from build123d import *

# Parameters (mm, degrees)
SKETCH3_W                    = 195
SKETCH3_H                    = 90
BASE_FLANGE1_DEPTH           = 0.76
EDGE_FLANGE1_STRIP_W         = 4.564
EDGE_FLANGE1_STRIP_H         = 0.76
EDGE_FLANGE1_STRIP_CUT_DEPTH = 90
EDGE_FLANGE1_DEPTH           = 90
EDGE_FLANGE2_STRIP_CUT_DEPTH = 90
EDGE_FLANGE2_DEPTH           = 90
EDGE_FLANGE3_STRIP_W         = 4.564
EDGE_FLANGE3_STRIP_H         = 0.76
EDGE_FLANGE3_STRIP_CUT_DEPTH = 90
EDGE_FLANGE3_DEPTH           = 90
EDGE_FLANGE6_DEPTH           = 124.238
EDGE_FLANGE7_DEPTH           = 124.238
CUT_EXTRUDE1_REACH           = 252.208


# Sheet-metal steps are written as plain solids
with BuildPart() as part:
    # Sketch3 → Base-Flange1 (new body)
    with BuildSketch(Plane(origin=(0, 0, 0), x_dir=(1, 0, 0), z_dir=(0, 1, 0))):
        with Locations((-97.5, 45)):
            Rectangle(SKETCH3_W, SKETCH3_H)
    extrude(amount=-BASE_FLANGE1_DEPTH)

    # Edge-Flange1 strip (across the edge) → Edge-Flange1 strip cut (cut)
    with BuildSketch(Plane(origin=(-195, 0, -90), x_dir=(1, 0, 0), z_dir=(0, 0, 1))):
        with Locations((-1.52, -0.38)):
            Rectangle(EDGE_FLANGE1_STRIP_W, EDGE_FLANGE1_STRIP_H)
    extrude(amount=EDGE_FLANGE1_STRIP_CUT_DEPTH, mode=Mode.SUBTRACT)

    # Edge-Flange1 section (across the edge) → Edge-Flange1 (add)
    with BuildSketch(Plane(origin=(-195, 0, -90), x_dir=(1, 0, 0), z_dir=(0, 0, 1))):
        with BuildLine():
            Line((-0.76, 0.762), (-0.76, 55))
            Line((-0.76, 55), (0, 55))
            Line((0, 55), (0, 0.762))
            ThreePointArc((0, 0.762), (0.223184633, 0.223184633), (0.762, 0))
            Line((0.762, 0), (0.762, -0.76))
            ThreePointArc((0.762, -0.76), (-0.314216521, -0.314216521), (-0.76, 0.762))
        make_face()
    extrude(amount=EDGE_FLANGE1_DEPTH)

    # Edge-Flange2 strip (across the edge) → Edge-Flange2 strip cut (cut)
    with BuildSketch(Plane(origin=(-195, 55, -90), x_dir=(-0.2588190451025146, -0.96592582628907, 0), z_dir=(0, 0, 1))):
        Polygon((-4.589327535, -2.016516504), (1.155922587, -0.477081374), (0.959220112, 0.257022254), (-4.786030009, -1.282412876), align=None)
    extrude(amount=EDGE_FLANGE2_STRIP_CUT_DEPTH, mode=Mode.SUBTRACT)

    # Edge-Flange2 section (across the edge) → Edge-Flange2 (add)
    with BuildSketch(Plane(origin=(-195, 55, -90), x_dir=(-0.2588190451025146, -0.96592582628907, 0), z_dir=(0, 0, 1))):
        with BuildLine():
            Line((-0.76, 0.993057734), (-0.76, 200))
            Line((-0.76, 200), (0, 200))
            Line((0, 200), (0, 0.993057734))
            ThreePointArc((0, 0.993057734), (0.298123791, 0.388522489), (0.959220112, 0.257022254))
            Line((0.959220112, 0.257022254), (1.155922587, -0.477081374))
            ThreePointArc((1.155922587, -0.477081374), (-0.164534895, -0.21442605), (-0.76, 0.993057734))
        make_face()
    extrude(amount=EDGE_FLANGE2_DEPTH)

    # Edge-Flange3 strip (across the edge) → Edge-Flange3 strip cut (cut)
    with BuildSketch(Plane(origin=(0, 0, 0), x_dir=(-1, 0, 0), z_dir=(0, 0, -1))):
        with Locations((-1.52, -0.38)):
            Rectangle(EDGE_FLANGE3_STRIP_W, EDGE_FLANGE3_STRIP_H)
    extrude(amount=EDGE_FLANGE3_STRIP_CUT_DEPTH, mode=Mode.SUBTRACT)

    # Edge-Flange3 section (across the edge) → Edge-Flange3 (add)
    with BuildSketch(Plane(origin=(0, 0, 0), x_dir=(-1, 0, 0), z_dir=(0, 0, -1))):
        with BuildLine():
            Line((-0.76, 0.762), (-0.76, 125))
            Line((-0.76, 125), (0, 125))
            Line((0, 125), (0, 0.762))
            ThreePointArc((0, 0.762), (0.223184633, 0.223184633), (0.762, 0))
            Line((0.762, 0), (0.762, -0.76))
            ThreePointArc((0.762, -0.76), (-0.314216521, -0.314216521), (-0.76, 0.762))
        make_face()
    extrude(amount=EDGE_FLANGE3_DEPTH)

    # Edge-Flange6 section (across the edge) → Edge-Flange6 (add)
    with BuildSketch(Plane(origin=(0, 0.762, 0.762), x_dir=(0, 0, -1), z_dir=(0, 1, 0))):
        with BuildLine():
            Line((-0.76, 0.762), (-0.76, 195.76))
            Line((-0.76, 195.76), (0, 195.76))
            Line((0, 195.76), (0, 0.762))
            ThreePointArc((0, 0.762), (0.223184633, 0.223184633), (0.762, 0))
            Line((0.762, 0), (0.762, -0.76))
            ThreePointArc((0.762, -0.76), (-0.314216521, -0.314216521), (-0.76, 0.762))
        make_face()
    extrude(amount=EDGE_FLANGE6_DEPTH)

    # Edge-Flange7 section (across the edge) → Edge-Flange7 (add)
    with BuildSketch(Plane(origin=(0, 125, -90.762), x_dir=(0, 0, 1), z_dir=(0, -1, 0))):
        with BuildLine():
            Line((-0.76, 0.762), (-0.76, 195.76))
            Line((-0.76, 195.76), (0, 195.76))
            Line((0, 195.76), (0, 0.762))
            ThreePointArc((0, 0.762), (0.223184633, 0.223184633), (0.762, 0))
            Line((0.762, 0), (0.762, -0.76))
            ThreePointArc((0.762, -0.76), (-0.314216521, -0.314216521), (-0.76, 0.762))
        make_face()
    extrude(amount=EDGE_FLANGE7_DEPTH)

    # Sketch29 → Cut-Extrude1 (cut, up to next)
    with BuildSketch(Plane.XY.offset(1.522), mode=Mode.PRIVATE) as cut_extrude1_sk1:
        Polygon((-195.76, 53.762), (-0.762, 0.762), (-195.76, 0.762), align=None)
    cut_extrude1_tool1 = extrude(cut_extrude1_sk1.sketch, amount=-CUT_EXTRUDE1_REACH, mode=Mode.PRIVATE) & part.part
    add(cut_extrude1_tool1.solids().sort_by_distance((-130.760667, 18.428667, 1.522))[0], mode=Mode.SUBTRACT)


solid = part.part
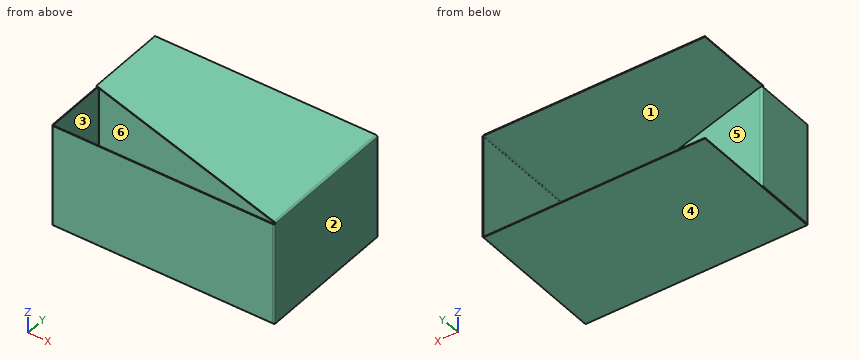
Design review of the part built by this model. Coordinates are the model's own, in mm. Face numbers are marked on the shaded views. A direction names the side the tool comes from. Round coordinates to 2 decimals unless told otherwise and drop trailing zeros. Write each loop counter-clockwise with the first axis right and the second up, starting at its lowest first coordinate (ties: lowest second). Pieces come first, ordered by that corner, then holes.
Item 1: For the marked faces 4, 5 and 6, list the 3-axis set-ups (+Z, -Z, +X, -X, +Y, -Y) from which the entire face can be reached by the end or side of a thin tool; tool diameter is ignored.
Item 2: Consider section B-B on x = -20. Give the boundary of the cut face in (y, z), and give its area (3 significant figures).
Item 3: For pin 1 Ø17 at (x, y) = (-124.5, 18.5) entering from +Z; pin 2 Ø1.5 at (x, z) = (-137, -80.5) entering from +Y; pin 3 Ø0.8 at (x, z) = (0, 0.5) entering from -Y, all flat-tipped, find the tip position at first contact; note any pin that passes through.
Item 4: Draft analysis for pull direction X (two halves, no side actions). For the marked faces 1, 2 and 3, state which applies: released by +X, released by -X, zero draft, split by the parting line, or undercut.
Item 5: Consider section A-A on y = 28. Give the boundary of the cut face in (x, z), and give its area (3 significant figures).
Item 6: Consider section D-D on y = 78.5. Give the boundary of the cut face in (x, z), and give its area (3 significant figures).
Item 7: Consider section C-C on z = -32. Give the boundary of the cut face in (x, y), and give its area (3 significant figures).
Item 8: Wall thickness on L1, parallel to Z at x = -166.5, y = 72; L2, parallel to Z at x = -174, y = 23.5; L3, parallel to Y at x = -120, z = -68.5: over which ranges is each line inside the solid? List them lowest first.
Check values:
1. face 4: -Z, +X, -X, +Y, -Y
1. face 5: +Y
1. face 6: none
2. outline: (-0.76, -90) - (0, -90) - (0, 0) - (-0.76, 0) - close; (0.76, -91.52) - (125, -91.52) - (125, -90.76) - (0.76, -90.76) - close; (5.99, 0.76) - (125, 0.76) - (125, 1.52) - (5.99, 1.52) - close; (8.11, -90) - (8.9, -90) - (8.9, 0) - (8.11, 0) - close
2. area: 324 mm2
3. pin 1: stops at z = -90.76
3. pin 2: stops at y = 40.45
3. pin 3: stops at y = 0.76
4. face 1: zero draft
4. face 2: released by +X
4. face 3: undercut
5. outline: (-195.76, -91.52) - (-0.76, -91.52) arc R1.52 ccw to (0.76, -90) - (0.76, 0) arc R1.52 ccw to (-0.76, 1.52) - (-100.98, 1.52) - (-100.98, 0.76) - (-0.76, 0.76) arc R0.76 cw to (0, 0) - (0, -90) arc R0.76 cw to (-0.76, -90.76) - (-195.76, -90.76) - close; (-195.76, -90) - (-195, -90) - (-195, 0) - (-195.76, 0) - close; (-94.23, -90) - (-91.3, -90) - (-91.3, 0) - (-94.23, 0) - close
5. area: 628 mm2
6. outline: (-195.76, -91.52) - (-0.76, -91.52) arc R1.52 ccw to (0.76, -90) - (0.76, 0) arc R1.52 ccw to (-0.76, 1.52) - (-195.76, 1.52) - (-195.76, 0.76) - (-0.76, 0.76) arc R0.76 cw to (0, 0) - (0, -90) arc R0.76 cw to (-0.76, -90.76) - (-195.76, -90.76) - close
6. area: 368 mm2
7. outline: (-195.76, 0.76) arc R1.52 ccw to (-194.24, -0.76) - (-0.76, -0.76) arc R1.52 ccw to (0.76, 0.76) - (0.76, 125) - (0, 125) - (0, 0.76) arc R0.76 cw to (-0.76, 0) - (-194.24, 0) arc R0.76 cw to (-195, 0.76) - (-195, 54.01) arc R0.76 cw to (-194.04, 54.74) - (-1.81, 3.24) - (-1.62, 3.97) - (-193.84, 55.48) arc R1.52 ccw to (-195.76, 54.01) - close
7. area: 437 mm2
8. L1: z = -91.52 to -90.76, 0.76 to 1.52
8. L2: z = -91.52 to -90.76
8. L3: y = -0.76 to 0, 34.9 to 35.69
